from build123d import *

# Parameters (mm, degrees)
ESQUISSE1_W        = 40.4
ESQUISSE1_H        = 20
BOSS_EXTRU_1_DEPTH = 1
ESQUISSE2_W        = 40.4
ESQUISSE2_H        = 20
ESQUISSE2_W_2      = 38.4
ESQUISSE2_H_2      = 18
BOSS_EXTRU_2_DEPTH = 2.1
CONG_1_R           = 1


with BuildPart() as part:
    # Esquisse1 → Boss.-Extru.1 (new body)
    with BuildSketch(Plane(origin=(0, 0, 0), x_dir=(1, 0, 0), z_dir=(0, 1, 0))):
        with Locations((-5.381395349, 0)):
            Rectangle(ESQUISSE1_W, ESQUISSE1_H)
    extrude(amount=BOSS_EXTRU_1_DEPTH)

    # Esquisse2 → Boss.-Extru.2 (add)
    with BuildSketch(Plane(origin=(0, 1, 0), x_dir=(1, 0, 0), z_dir=(0, 1, 0))):
        with Locations((-5.381395349, 0)):
            Rectangle(ESQUISSE2_W, ESQUISSE2_H)
        with Locations((-5.381395349, 0)):
            Rectangle(ESQUISSE2_W_2, ESQUISSE2_H_2, mode=Mode.SUBTRACT)
    extrude(amount=BOSS_EXTRU_2_DEPTH)

    # Congé1
    cong_1_edges = [part.edges().sort_by_distance(p)[0] for p in [
        (-5.381395349, 0, -10),
        (14.818604651, 0, 0),
        (-5.381395349, 0, 10),
        (-25.581395349, 0, 0),
        (-25.581395349, 1.55, -10),
        (14.818604651, 1.55, -10),
        (14.818604651, 1.55, 10),
        (-25.581395349, 1.55, 10),
    ]]
    fillet(cong_1_edges, radius=CONG_1_R)


solid = part.part
Here's how the part is built. I have some questions about the finished solid (model axes, mm). A direction names the side the tool comes from. Coordinates: 2 decimals unless noted, no trailing zeros. Write each loop counter-clockwise with the first axis right and the second up, starting at its lowest first coordinate (ties: lowest second). Pieces come first, ordered by that corner, then holes.
1) If we section it at C-C (z = 6.75): List the corners of the cut face in (x, y) for me, plus the area to 3 significant figures.
Filled in:
outline: (-25.58, 1) arc R1 ccw to (-24.58, 0) - (13.82, 0) arc R1 ccw to (14.82, 1) - (14.82, 3.1) - (13.82, 3.1) - (13.82, 1) - (-24.58, 1) - (-24.58, 3.1) - (-25.58, 3.1) - close
area: 44.2 mm2
2) I'm going to push a flat-ended pin straight in: pin 1 (8 mm diameter, centred on x = -5.5, z = 4, fed in from +Y). Where does the tip first touch, or does it pass through?
Filled in:
pin 1: stops at y = 1
3) Thinking about a two-plate mould opening in Z: for faces 3 (the face through (13.819, 2, 0)), 4 (the face through (-25.581, 2, 0)), 5 (the face through (14.52, 2.06, 9.71)), which applies, +Z half, -Z half, draft (parallel to the pull), parting line (faces both ways), or undercut?
Filled in:
face 3: undercut
face 4: draft
face 5: +Z half
4) Which directions (+Z, -Z, +X, -X, +Y, -Y) give clear straight access to the entire face, cutting with the end or side of a thin tool? Please do faces 1 (the face through (-6, 2, -10)), 2 (the face through (-6, 2, 9)).
Filled in:
face 1: -Z, +X, -X, +Y, -Y
face 2: +Y
5) If we section it at A-A (y = 2.2): List the corners of the cut face in (x, z) for me, plus the area to 3 significant figures.
Filled in:
outline: (-25.58, -9) arc R1 ccw to (-24.58, -10) - (13.82, -10) arc R1 ccw to (14.82, -9) - (14.82, 9) arc R1 ccw to (13.82, 10) - (-24.58, 10) arc R1 ccw to (-25.58, 9) - close; hole (-24.58, -9) - (13.82, -9) - (13.82, 9) - (-24.58, 9) - close
area: 116 mm2
6) If I drill on line 1 (Z direction, x = -14, y = 2.95); line 2 (X direction, y = 2.4, z = -1.75); line 3 (Y direction, x = -11, z = 8.75), over which ranges is the centre line in solid material (lowest first)?
Filled in:
line 1: z = -10 to -9, 9 to 10
line 2: x = -25.58 to -24.58, 13.82 to 14.82
line 3: y = 0 to 1
7) If we section it at B-B (x = -14.5): List the corners of the cut face in (y, z) for me.
Filled in:
outline: (0, -9) arc R1 ccw to (1, -10) - (3.1, -10) - (3.1, -9) - (1, -9) - (1, 9) - (3.1, 9) - (3.1, 10) - (1, 10) arc R1 ccw to (0, 9) - close
